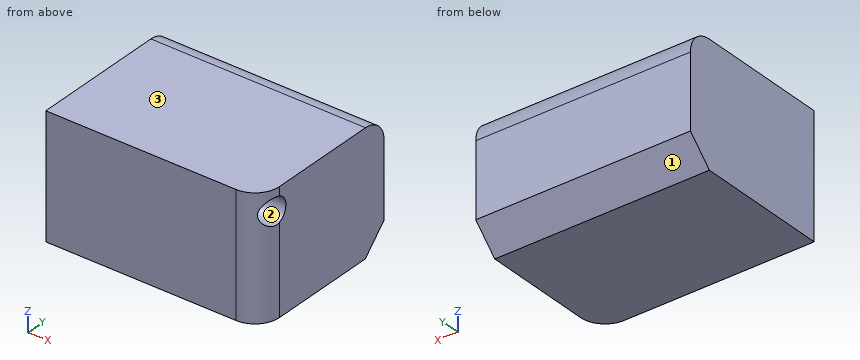
```python
from build123d import *

# Parameters (mm, degrees)
F0_W        = 44.6331575513
F0_H        = 33.0944694579
F1_DEPTH    = 25.4
F2_R        = 5
F3_SIZE     = 5.08
F4_R        = 2.7454645763
F5_DEPTH    = 25.4
F6_T1_DEPTH = 50.8


# Not quite as in the source:
# - a fillet or chamfer that OpenCascade refuses, or shapes differently, is made with other operations: its cross-section is extruded or revolved along the edge and cut away or added


with BuildPart() as f1:
    # F0 (on Top) → F1 (new body)
    with BuildSketch(Plane.XY):
        with Locations((22.3165787756, -16.5472347289)):
            Rectangle(F0_W, F0_H)
    extrude(amount=F1_DEPTH)

    # F2
    f2_edges = [f1.edges().sort_by_distance(p)[0] for p in [
        (22.316579, 0, 25.4),
    ]]
    fillet(f2_edges, radius=F2_R)

    # F3
    f3_edges = [f1.edges().sort_by_distance(p)[0] for p in [
        (22.316579, 0, 0),
    ]]
    chamfer(f3_edges, length=F3_SIZE)

    # F4 (on face) → F5 (cut)
    with BuildSketch(Plane.YZ.offset(44.6331575513)):
        with Locations((-29.0195755661, 21.0298281163)):
            Circle(F4_R)
    extrude(amount=-F5_DEPTH, mode=Mode.SUBTRACT)

    # F6: fillet of radius 5.08 on 1 edges, made by hand

    # F6_s2 → F6_t1 (cut)
    with BuildSketch(Plane.XY.offset(-12.7)):
        with BuildLine():
            ThreePointArc((44.6331575513, -28.0144694579), (43.1452599997, -31.6065719063), (39.5531575513, -33.0944694579))
            Line((39.5531575513, -33.0944694579), (44.6331575513, -33.0944694579))
            Line((44.6331575513, -33.0944694579), (44.6331575513, -28.0144694579))
        make_face()
    extrude(amount=F6_T1_DEPTH, mode=Mode.SUBTRACT)


solid = f1.part
```
Can you work these out from the model? Positions are in its coordinate system, mm. Face numbers are marked on the shaded views. Give positions to 0.01 mm unless a question says otherwise; leave off trailing zeros. Write each loop counter-clockwise with the first axis right and the second up, starting at its lowest first coordinate (ties: lowest second). Pieces come first, ordered by that corner, then holes. Notation, with made-up numbers: (31, -29) - (81, -29) arc R15 ccw to (81, -20) - close; hole circle Ø1 at (47, 50). An arc over 180 degrees is marked (long way). Write item = value, one per line. Start each with the question number.
1. Thinking about a two-plate mould opening in Z: for the marked faces 1, 2 and 3, which applies, released by +Z, released by -Z, zero draft, split by the parting line, or undercut?
2. Please list where these lines run through material, in increasing order: line 1 (X direction, y = -30.5, z = 10.75); line 2 (Y direction, x = 8, z = 3.5); line 3 (Z direction, x = 18, y = -3).
3. Imagine slicing it at C-C (x = 18). Please give me the cut outline in (y, z), and give its area (3 significant figures).
4. For pin 1 (6 mm diameter, centred on y = -29.5, z = 21.5, fed in from +X), with a flat end and sliding along its axis, tell me the tip position at first contact or that it passes through.
5. Imagine slicing it at B-B (x = 29.5). Please give me the cut outline in (y, z), and give its area (3 significant figures).
6. Imagine slicing it at D-D (y = -2.5). Please give me the cut outline in (x, z).
7. Imagine slicing it at A-A (z = 2.25). Please give me the cut outline in (x, y).
Worked answers:
q1.face_1 = released by -Z
q1.face_2 = undercut
q1.face_3 = released by +Z
q2.line_1 = 0 to 43.98
q2.line_2 = -33.09 to -1.58
q2.line_3 = 2.08 to 24.98
q3.outline = (-33.09, 0) - (-5.08, 0) - (0, 5.08) - (0, 20.4) arc R5 ccw to (-5, 25.4) - (-33.09, 25.4) - close
q3.area = 822 mm2
q4.pin_1 = 44.63
q5.outline = (-33.09, 0) - (-5.08, 0) - (0, 5.08) - (0, 20.4) arc R5 ccw to (-5, 25.4) - (-33.09, 25.4) - close; hole circle Ø5.49 at (-29.02, 21.03)
q5.area = 799 mm2
q6.outline = (0, 2.58) - (44.63, 2.58) - (44.63, 24.73) - (0, 24.73) - close
q7.outline = (0, -33.09) - (39.55, -33.09) arc R5.08 ccw to (44.63, -28.01) - (44.63, -2.83) - (0, -2.83) - close
